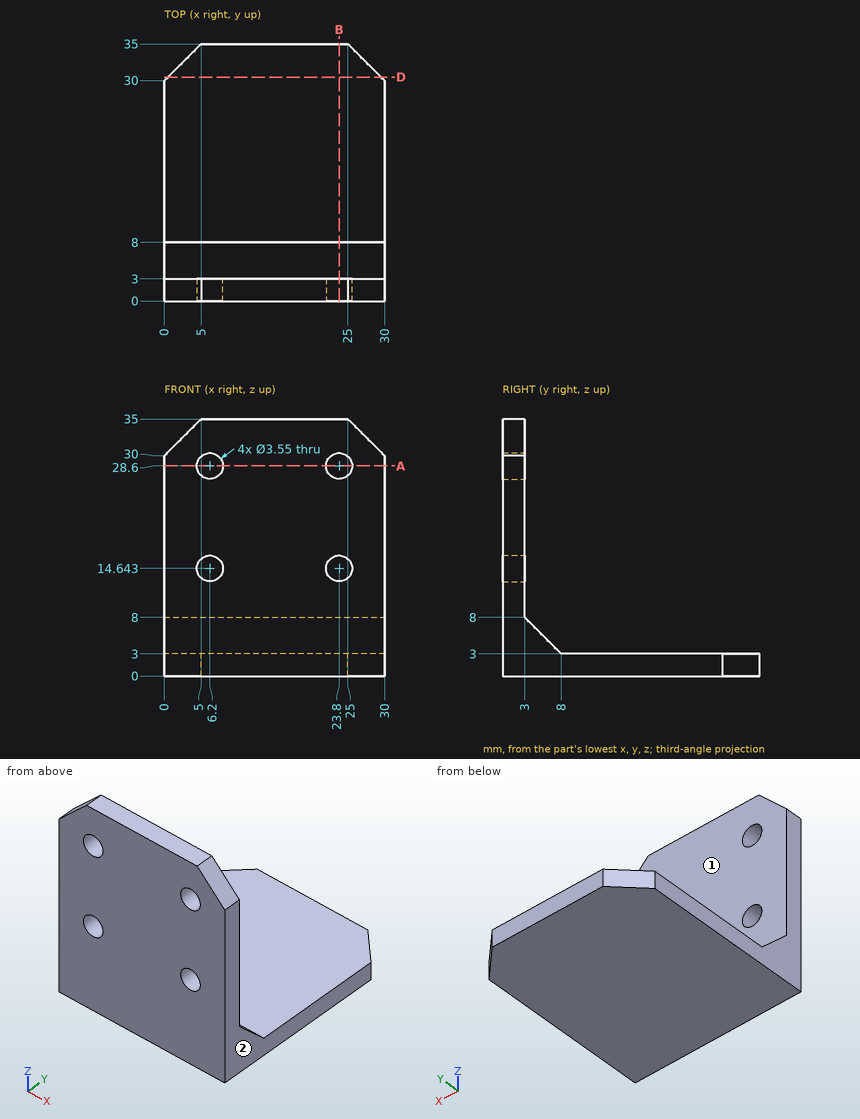
The figure shows three views and two pictorial views of one solid part (mm, origin at its lowest corner). Answer the questions. A direction names the side the tool comes from. Give positions to 0.01 mm unless a question says otherwise; leave off trailing zeros. Write each loop counter-clockwise with the first axis right and the second up, starting at its lowest first coordinate (ties: lowest second). Pieces come first, ordered by that corner, then holes. Notation, with made-up numbers: M 44,45 L 57,45 A19 cw 57,70 Z; hole C -16.75,-10 d8. An arc over 180 degrees is marked long. One line per item, written item: value. Start each with the question number.
(1) A tool of negligible diameter and unlimited length cuts with its end or side. For the marked faces 1 and 2, from which of +Z, -Z, +X, -X, +Y, -Y can it reach the whole face along a straight path? Write none if from no direction.
(2) Find the intervals of material crossed by line 1 (Z direction, x = 23.8, y = 2.3) (1 decimal); line 2 (X direction, y = 1, z = 28); line 3 (Y direction, x = 26, z = 31), in increasing order.
(3) Flat-ended cylindrical pins translate along their axes: pin 1 Ø4.5 at (x, z) = (23.8, 14.64) entering from +Y; pin 2 Ø8 at (x, z) = (10, 9.5) entering from +Y; pin 3 Ø10 at (x, y) = (7, 17) entering from +Z. Find the tip coordinate at first contact, or state that the pin passes through.
(4) Find section D-D (y = 30.5). Determine the outline of the cut face in (x, z).
(5) Find section B-B (x = 23.8). Give the number of separate pieces and of enclosed holes in the cut face, plus the area to 3 significant figures.
(6) Find section A-A (z = 28.6). Determine the outline of the cut face in (x, y) (1 decimal).
Results below:
1. face 1: +Z, +X, -X, +Y
1. face 2: +Z, -Z, +X, +Y, -Y
2. line 1: z = 0 to 12.9, 16.4 to 26.8, 30.4 to 35
2. line 2: x = 0 to 4.53, 7.87 to 22.13, 25.47 to 30
2. line 3: y = 0 to 3
3. pin 1: stops at y = 3
3. pin 2: stops at y = 5.5
3. pin 3: stops at z = 3
4. outline: M 0.5,0 L 29.5,0 L 29.5,3 L 0.5,3 Z
5. separate pieces: 3
5. enclosed holes: 0
5. area: 192 mm^2
6. outline: M 0,0 L 4.4,0 L 4.4,3 L 0,3 Z; M 8,0 L 22,0 L 22,3 L 8,3 Z; M 25.6,0 L 30,0 L 30,3 L 25.6,3 Z
